Design review of the part shown in the three views and the two pictorial views. Dimensions are in mm from the part's minimum x, y and z. Round coordinates to 2 decimals unless told otherwise and drop trailing zeros. Write each loop counter-clockwise with the first axis right and the second up, starting at its lowest first coordinate (ties: lowest second). Pieces come first, ordered by that corner, then holes. Notation, with made-up numbers: (-28.75, 56.25) - (30.25, 56.25) arc R32 cw to (30.25, 95.25) - close; hole circle Ø3 at (-34, 32.5). An arc over 180 degrees is marked (long way). Use one line per item in the form item = value.
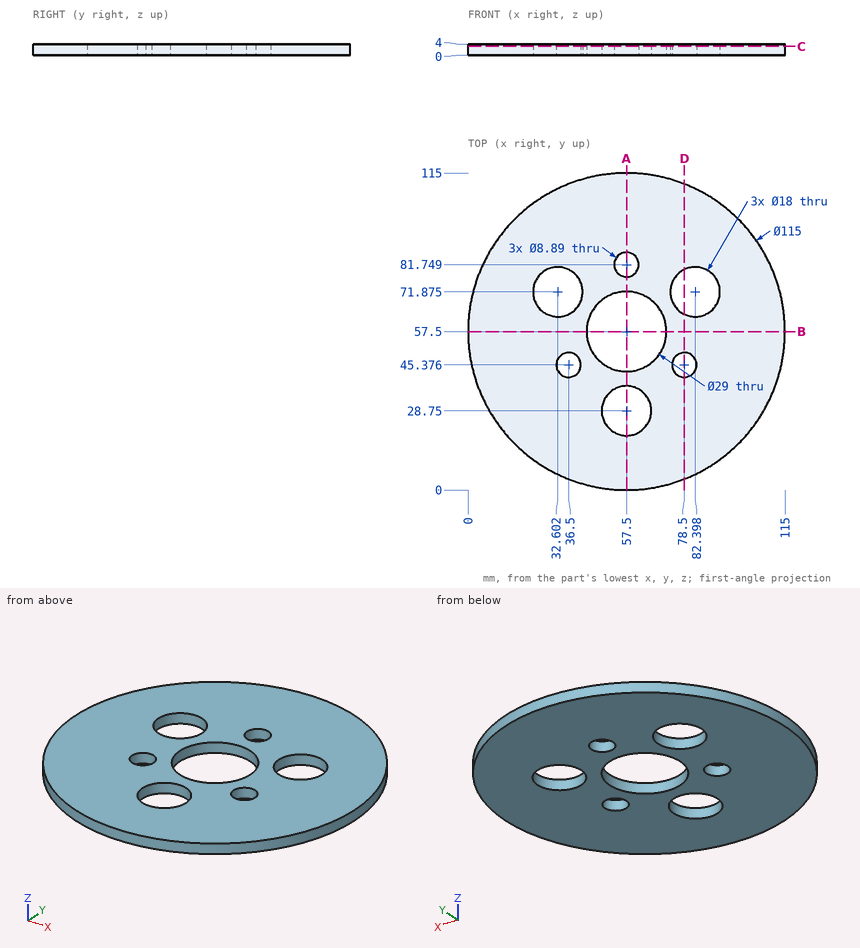
(1) Add section A-A on x = 57.5. Write out the cut boundary in (y, z).
Geometry results:
outline = (0, 0) - (19.75, 0) - (19.75, 4) - (0, 4) - close; (37.75, 0) - (43, 0) - (43, 4) - (37.75, 4) - close; (72, 0) - (77.3, 0) - (77.3, 4) - (72, 4) - close; (86.19, 0) - (115, 0) - (115, 4) - (86.19, 4) - close
(2) Add section D-D on x = 78.5. Write out the cut boundary in (y, z), then the cut area to 3 significant figures.
Geometry results:
outline = (3.97, 0) - (40.93, 0) - (40.93, 4) - (3.97, 4) - close; (49.82, 0) - (63.76, 0) - (63.76, 4) - (49.82, 4) - close; (79.99, 0) - (111.03, 0) - (111.03, 4) - (79.99, 4) - close
area = 328 mm2
(3) Insertion check: P1, Ø16, axis at x = 32.6, y = 71.88, coming from the +Z side; P2, Ø8, axis at x = 43, y = 99, coming from the -Z side; P3, Ø2, axis at x = 28, z = 2.5, coming from the -Y side; P4, Ø2, axis at y = 22, z = 3, coming from the +X side. Each pin has a flat end and moves straight along its axis. Give the tip position at first contact, or say it passes through.
Geometry results:
P1 = through
P2 = 0
P3 = 7.56
P4 = 103.5
(4) To check wall thickness, follow L1, parallel to Y at x = 57.5, z = 1.65; L2, parallel to Y at x = 63, z = 2.25 (1 decimal); L3, parallel to X at y = 48, z = 3.2 (1 decimal). State the ranges of each line that lie inside material, in increasing order.
Geometry results:
L1 = 0 to 19.75, 37.75 to 43, 72 to 77.3, 86.19 to 115
L2 = 0.3 to 21.6, 35.9 to 44.1, 70.9 to 114.7
L3 = 0.8 to 32.9, 40.1 to 46.5, 68.5 to 74.9, 82.1 to 114.2
(5) Add section C-C on z = 3.15. Count the separate pieces of the cut face and the enclosed holes in it, then the cut area to 3 significant figures.
Geometry results:
separate_pieces = 1
enclosed_holes = 7
area = 8,780 mm2
(6) Add section B-B on y = 57.5. Write out the cut boundary in (x, z).
Geometry results:
outline = (0, 0) - (43, 0) - (43, 4) - (0, 4) - close; (72, 0) - (115, 0) - (115, 4) - (72, 4) - close
